Design review of the part built by this model. Coordinates are the model's own, in mm. Face numbers are marked on the shaded views. Give positions to 0.01 mm unless a question says otherwise; leave off trailing zeros. Loops run counter-clockwise (first coordinate to the right, second up) from the corner with the lowest first, then second, coordinate; pieces in that order, holes last. Notation, with made-up numbers: M -4.5,37.25 L 17.5,37.25 A35 ccw 17.5,70.25 Z; hole C 30,55 d8. An arc over 180 degrees is marked long. Use CSV: the item, a comma, the result in double quotes.
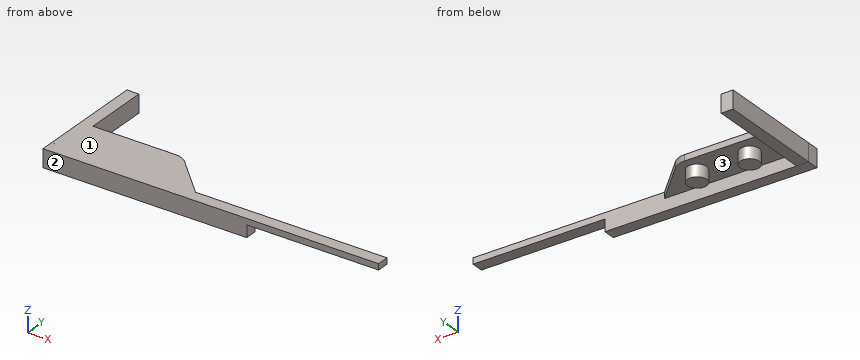
Autodesk Inventor part; units mm, degrees
ref_plane "YZ Plane" through (0, 0, 0) normal (1, 0, 0) x (0, 1, 0)
ref_plane "XZ Plane" through (0, 0, 0) normal (0, 1, 0) x (-1, 0, 0)
ref_plane "XY Plane" through (0, 0, 0) normal (0, 0, 1) x (1, 0, 0)
sketch "Sketch1" plane through (0, 0, 0) normal (0, 0, 1) x (1, 0, 0)
  line L0 (0, 0) -> (140, 0)
  line L1 (140, 0) -> (140, 60) construction
  line L2 (140, 60) -> (0, 60) construction
  line L3 (0, 60) -> (0, 0) construction
  line L4 (0, 45) -> (15, 60)
  line L5 (0, 45) -> (21.2132, 45) construction
  line L6 (0, 45) -> (140, 45) construction
  line L7 (140, 45) -> (125, 60)
  line L8 (140, 45) -> (161.2132, 45) construction
  line L9 (0, 0) -> (0, 45)
  line L10 (140, 0) -> (140, 45)
  line L11 (125, 60) -> (15, 60)
  line L12 (0, 0) -> (140, 0)
  line L13 (140, 0) -> (140, 5)
  line L14 (140, 5) -> (0, 5) construction
  line L15 (0, 5) -> (0, 0)
  line L16 (0, 0) -> (5, 0)
  line L17 (5, 0) -> (5, 50) construction
  line L18 (5, 50) -> (0, 50) construction
  line L19 (0, 50) -> (0, 0) construction
  line L20 (140, 0) -> (135, 0) construction
  line L21 (135, 0) -> (135, 50) construction
  line L22 (135, 50) -> (140, 50) construction
  line L23 (140, 50) -> (140, 0) construction
  line L24 (0, 45) -> (30, 45)
  line L25 (140, 45) -> (30, 45)
  line L26 (85, 45) -> (100, 60)
  line L27 (140, 45) -> (34.9105, 45)
  line L28 (34.9105, 0) -> (140, 0)
  line L29 (140, 0) -> (140, 45)
  line L30 (0, 0) -> (10, 0)
  line L31 (10, 0) -> (10, 45) construction
  line L32 (10, 45) -> (0, 45)
  line L33 (0, 45) -> (0, 0)
  line L34 (10, 5) -> (25.8293, 5) construction
  circle A0 centre (81.8934, 52.5) radius 7.5 construction
  line L35 (81.8934, 52.5) -> (39.467, 10.0736) construction
  line L36 (81.8934, 52.5) -> (141.8934, 52.5) construction
  circle A1 centre (39.467, 10.0736) radius 7.5
  circle A2 centre (17.5, 10.0736) radius 7.5
  line L37 (17.5, 10.0736) -> (39.467, 10.0736) construction
  line L38 (17.5, 10.0736) -> (59.9264, 52.5) construction
  line L39 (17.5, 10.0736) -> (77.5, 10.0736) construction
  circle A3 centre (59.9264, 52.5) radius 7.5 construction
  line L40 (59.9264, 52.5) -> (81.8934, 52.5) construction
  circle A4 centre (52.4264, 45) radius 7.5 construction
  circle A5 centre (74.3934, 45) radius 7.5 construction
  line L41 (12.1967, 15.3769) -> (47.1231, 50.3033) construction
  line L42 (57.7297, 39.6967) -> (22.8033, 4.7703) construction
  line L43 (34.1637, 15.3769) -> (69.0901, 50.3033) construction
  line L44 (79.6967, 39.6967) -> (44.7703, 4.7703) construction
  circle A6 centre (52.4264, 45) radius 8
  circle A7 centre (74.3934, 45) radius 8
  line L45 (52.4264, 45) -> (74.3934, 45)
  line L46 (46.7696, 50.6569) -> (41.1127, 45)
  line L47 (46.7696, 50.6569) -> (54.7696, 50.6569) construction
  line L48 (79.0022, 38.461) -> (36.7044, 38.461) construction
  line L49 (52.4264, 53) -> (93, 53)
  circle A8 centre (17.5, 10.0736) radius 4
  circle A9 centre (39.467, 10.0736) radius 4
  line L50 (0, 0) -> (140, 0)
  line L51 (140, 0) -> (140, -5)
  line L52 (140, -5) -> (0, -5)
  line L53 (0, -5) -> (0, 0)
  line L54 (0, 45) -> (5, 45)
  line L55 (5, 45) -> (5, -0.0081)
  line L56 (5, -0.0081) -> (0, -0.0081)
  line L57 (0, -0.0081) -> (0, 45)
  line L58 (17.5, 17.5736) -> (5, 17.5736)
  line L59 (44.7703, 15.3769) -> (60.1472, 0)
  line L60 (39.467, 17.5736) -> (17.5, 17.5736)
  line L61 (85, 45) -> (85, 0)
  line L62 (85, 0) -> (85, -5)
  point P0 (43.467, 0)
  dimension "d19" = 16
  dimension "d0" = 140
  dimension "d1" = 60
  dimension "d2" = 45
  dimension "d3" = 15
  dimension "d4" = 135
  dimension "d5" = 5
  dimension "d6" = 5
  dimension "d7" = 5
  dimension "d8" = 25
  dimension "d9" = 10
  dimension "d10" = 60
  dimension "d11" = 135
  dimension "d12" = 15
  dimension "d13" = 15
  dimension "d14" = 60
  dimension "d15" = 45
  dimension "d16" = 15
  dimension "d17" = 15
  dimension "d18" = 16
  dimension "d20" = 135
  dimension "d21" = 8
  dimension "d22" = 8
  dimension "d23" = 5
  dimension "d24" = 5
extrude "Extrusion1" add sketch "Sketch1" against normal blind 7.5 contours L9 L24 L55 L0 | L0 L62 L52 L53 L56 L55 | A8 | A9
extrude "Extrusion2" add sketch "Sketch1" against normal blind 2.5 contours A2 | L55 L58 L60 A1 L59 L0 | L62 L0 L51 L52 | A1
properties part number "Basseipt"
(1) The part is to be moulded in two halves that separate along Y. For the marked faces 1, 2 and 3, say which applies: released by +Y, released by -Y, zero draft, split by the parting line, or undercut.
A:
face 1,"zero draft"
face 2,"released by -Y"
face 3,"undercut"
(2) We need section C-C on y = -1.5. State the section outline as (x, z) points, then the cut area to 3 significant figures.
A:
outline,"M 0,-7.5 L 85,-7.5 L 85,-2.5 L 140,-2.5 L 140,0 L 0,0 Z"
area,"775 mm²"
(3) Clearance check with flat-ended pins moving along their axes: P1, Ø3, axis at y = 19, z = -5.5, coming from the +X side; P2, Ø1.2, axis at x = 28, z = -1, coming from the +Y side; P3, Ø3, axis at x = 104.5, z = -5, coming from the +Y side; P4, Ø2.5, axis at y = -3, z = -4, coming from the +X side. State where each tip first meets the part, or that it passes through.
A:
P1,"x = 5"
P2,"y = 17.57"
P3,"through"
P4,"x = 85"
(4) We need section B-B on x = 25.5. State the section outline as (y, z) points.
A:
outline,"M -5,-7.5 L 0,-7.5 L 0,-2.5 L 17.57,-2.5 L 17.57,0 L -5,0 Z"
(5) Wall thickness on line 1 along Y through (x, z) = (39, -2.75); line 2 along X through (y, z) = (11, -6.25); line 3 along X through (y, z) = (40, -4.5): over which ranges is each line inside the solid? List them lowest first. Write a range as [from, to].
A:
line 1,"[-5, 0], [6.1, 14.05]"
line 2,"[0, 5], [13.61, 21.39], [35.58, 43.36]"
line 3,"[0, 5]"
(6) We need section D-D on y = 19.5. State the section outline as (x, z) points.
A:
outline,"M 0,-7.5 L 5,-7.5 L 5,0 L 0,0 Z"
